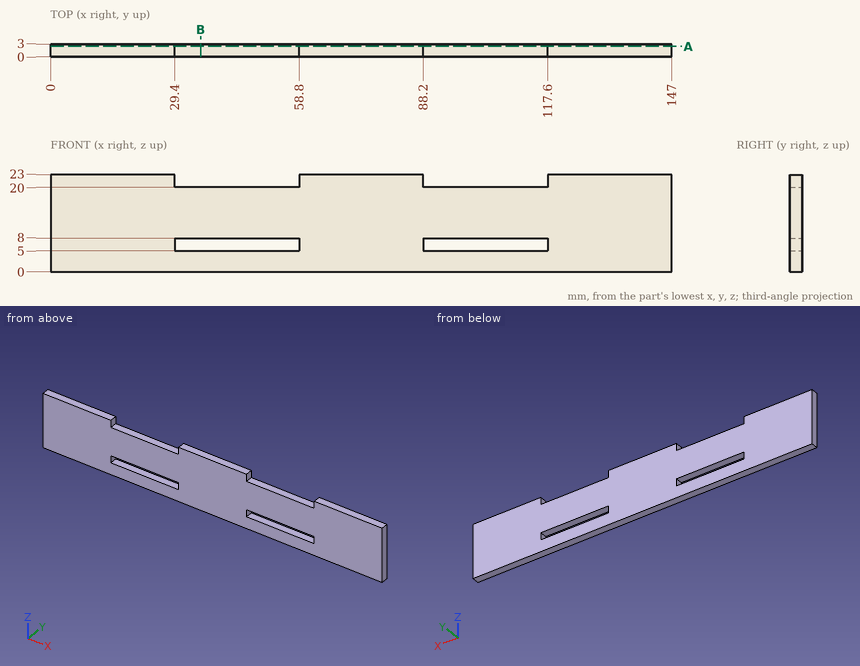
Here's the drawing with two shaded views (mm, measured from the low corner). I have some questions. Round coordinates to 2 decimals unless told otherwise and drop trailing zeros. Order: outer loops, then holes, each group sorted by start corner. A loop starts at its lowest first (then second) coordinate and runs counter-clockwise, first axis right, second up. Notation, with made-up numbers: (65, 83.25) -> (115, 83.25) arc R26 cw to (115, 119.25) -> close; hole circle Ø3 at (42, 28). An arc over 180 degrees is marked (long way). Use a Markdown table: item, result. Add a question column.
(1) Suppose I cut it at A-A, the plane y = 2.45. Please give me the cut outline in (x, z).
(2) I need wall thicknesses on line 1 along X through (y, z) = (2.9, 5.25); line 2 along Z through (x, y) = (30.5, 1). Which ranges of each line are inside material? Lowest first, please.
(3) Suppose I cut it at B-B, the plane x = 35.5. Please give me the cut outline in (y, z), and give its area (3 significant figures).
(4) For pin 1 Ø0.9 at (x, y) = (106, 1) entering from +Z, with a flat end and sliding along its axis, tell me the tip position at first contact or that it passes through.
Verdict:
| question | item | result |
|---|---|---|
| 1 | outline | (0, 0) -> (147, 0) -> (147, 23) -> (117.6, 23) -> (117.6, 20) -> (88.2, 20) -> (88.2, 23) -> (58.8, 23) -> (58.8, 20) -> (29.4, 20) -> (29.4, 23) -> (0, 23) -> close; hole (29.4, 5) -> (58.8, 5) -> (58.8, 8) -> (29.4, 8) -> close; hole (88.2, 5) -> (117.6, 5) -> (117.6, 8) -> (88.2, 8) -> close |
| 2 | line 1 | 0 to 29.4, 58.8 to 88.2, 117.6 to 147 |
| 2 | line 2 | 0 to 5, 8 to 20 |
| 3 | outline | (0, 0) -> (3, 0) -> (3, 5) -> (0, 5) -> close; (0, 8) -> (3, 8) -> (3, 20) -> (0, 20) -> close |
| 3 | area | 51.0 mm2 |
| 4 | pin 1 | z = 20 |
